Part model, mm, in its own coordinate system. A direction names the side the tool comes from. Give positions to 0.01 mm unless a question says otherwise; leave off trailing zeros. Loops run counter-clockwise (first coordinate to the right, second up) from the corner with the lowest first, then second, coordinate; pieces in that order, holes last. Notation, with made-up numbers: (-4, 66) -> (19, 66) arc R15 cw to (19, 89) -> close; hole circle Ø8 at (3, 84). An arc over 180 degrees is marked (long way). One line per question, with ' | ' between items.
```python
from build123d import *

# Parameters (mm, degrees)
SKETCH_1_R               = 14
SKETCH_1_R_2             = 11.8
EXTRUDE_1_DEPTH          = 14
SKETCH_2_R               = 14
EXTRUDE_2_DEPTH          = 4
CHAMFER_1_SIZE           = 1
CHAMFER_1_SIZE2          = 10
SKETCH_3_R               = 4
EXTRUDE_3_DEPTH          = 3
SKETCH_4_R               = 3
EXTRUDE_4_DEPTH          = 11
SKETCH_5_W               = 6.079740031
SKETCH_5_H               = 11.892824797
SKETCH_5_W_2             = 4.533139496
SKETCH_5_H_2             = 13.012776908
CUT_EXTRUDE_1_DEPTH      = 3
CUT_EXTRUDE_2_DEPTH      = 4
PATTERN_CIRCULAR_1_COUNT = 5


with BuildPart() as part:
    # Эскиз1 → Бобышка-Вытянуть1 (new body)
    with BuildSketch(Plane(origin=(0, 0, 0), x_dir=(1, 0, 0), z_dir=(0, 1, 0))):
        Circle(SKETCH_1_R)
        Circle(SKETCH_1_R_2, mode=Mode.SUBTRACT)
    extrude(amount=EXTRUDE_1_DEPTH)

    # Эскиз2 → Бобышка-Вытянуть2 (add)
    with BuildSketch(Plane(origin=(0, 14, 0), x_dir=(1, 0, 0), z_dir=(0, 1, 0))):
        Circle(SKETCH_2_R)
    extrude(amount=EXTRUDE_2_DEPTH)

    # Фаска1
    chamfer_1_edges = [part.edges().sort_by_distance(p)[0] for p in [
        (-14, 18, 0),
    ]]
    chamfer_1_side = [part.faces().sort_by_distance(p)[0] for p in [
        (-14, 9, 0),
    ]]
    chamfer(chamfer_1_edges, length=CHAMFER_1_SIZE, length2=CHAMFER_1_SIZE2, reference=chamfer_1_side[0])

    # Эскиз3 → Бобышка-Вытянуть3 (add)
    with BuildSketch(Plane(origin=(0, 18, 0), x_dir=(1, 0, 0), z_dir=(0, 1, 0))):
        Circle(SKETCH_3_R)
    extrude(amount=EXTRUDE_3_DEPTH)

    # Эскиз4 → Бобышка-Вытянуть4 (add)
    with BuildSketch(Plane(origin=(0, 21, 0), x_dir=(1, 0, 0), z_dir=(0, 1, 0))):
        Circle(SKETCH_4_R)
    extrude(amount=EXTRUDE_4_DEPTH)

    # Эскиз5 → Вырез-Вытянуть1 (cut)
    with BuildSketch(Plane(origin=(0, 21, 0), x_dir=(1, 0, 0), z_dir=(0, 1, 0))):
        with Locations((-6.539870016, -0.426648424)):
            Rectangle(SKETCH_5_W, SKETCH_5_H)
        with Locations((5.766569748, 0.133327632)):
            Rectangle(SKETCH_5_W_2, SKETCH_5_H_2)
    extrude(amount=-CUT_EXTRUDE_1_DEPTH, mode=Mode.SUBTRACT)

    # Эскиз6 → Вырез-Вытянуть2 (cut)
    with BuildSketch(Plane(origin=(0, 18, 0), x_dir=(1, 0, 0), z_dir=(0, 1, 0))):
        with BuildLine():
            Line((-3.5, -7.5), (-3.5, -15.705995079))
            Line((-3.5, -15.705995079), (3.5, -15.705995079))
            Line((3.5, -15.705995079), (3.5, -7.5))
            ThreePointArc((3.5, -7.5), (0, -4), (-3.5, -7.5))
        make_face()
    cut_extrude_2 = extrude(amount=-CUT_EXTRUDE_2_DEPTH, mode=Mode.SUBTRACT)

    # Круговой массив1: Вырез-Вытянуть2 ×5 about axis
    pattern_circular_1_axis = Axis((0, 0, 0), (0, 1, 0))
    for i in range(1, PATTERN_CIRCULAR_1_COUNT):
        add(cut_extrude_2.rotate(pattern_circular_1_axis, i * 360 / PATTERN_CIRCULAR_1_COUNT), mode=Mode.SUBTRACT)


solid = part.part
```
1) Drill centre lines: line 1 (X direction, y = 4, z = 0); line 2 (Z direction, x = 6.25, y = 9). Where is each one in solid material? Low to high.
Found:
line 1: -14 to -11.8, 11.8 to 14 | line 2: -12.53 to -10.01, 10.01 to 12.53
2) Saw through at D-D (y = 27.5). Give the cut face in (x, z).
Found:
outline: circle Ø6 at (0, 0)
3) Saw through at A-A (y = 3.5). Give the cut face in (x, z).
Found:
outline: circle Ø28 at (0, 0); hole circle Ø23.6 at (0, 0)
4) Tool access for faces 1 (the cylindrical face through (-11.79, 6.9, -0.52)), 2 (the flat face through (-9.04, 15.81, -6.49)), 3 (the cylindrical face through (-3, 26, 0)): list every direction of +Z, -Z, +X, -X, +Y, -Y with a clear straight run to the whole face (end or side of a thin tool).
Found:
face 1: -Y | face 2: -Z, +Y | face 3: +Y
5) Pin check, flat tips, straight feed: P1, Ø1.5, axis at x = 11, y = 13.5, coming from the -Z side; P2, Ø5, axis at x = -13, z = 2.5, coming from the +Y side; P3, Ø3.5, axis at x = 13, z = 4, coming from the +Y side; P4, Ø6, axis at y = 26.5, z = 7, coming from the +X side. Stop position of each tip, or through.
Found:
P1: z = -9.54 | P2: y = 17.2 | P3: y = 14 | P4: through
6) Saw through at B-B (x = 4.5). State how many separate pieces and enclosed holes the cut face has, and give its area (3 significant figures).
Found:
separate pieces: 3 | enclosed holes: 0 | area: 109 mm2
7) Pull direction Z, two halves, no side cores. Call faces 4 (the cylindrical face through (0, 19, -4)), 5 (the conical face through (-5.312, 17.507, 7.178)), 6 (the flat face through (-3.3, 15.8, -10.5)): pulls with the +Z half, pulls with the -Z half, needs draft (parallel to the pull), parting line crosses it, or undercut.
Found:
face 4: pulls with the -Z half | face 5: pulls with the +Z half | face 6: undercut
